Autodesk Inventor part; units mm, degrees
ref_plane "YZ Plane" through (0, 0, 0) normal (1, 0, 0) x (0, 1, 0)
ref_plane "XZ Plane" through (0, 0, 0) normal (0, 1, 0) x (-1, 0, 0)
ref_plane "XY Plane" through (0, 0, 0) normal (0, 0, 1) x (1, 0, 0)
sketch "Sketch1" plane through (0, 0, 0) normal (0, 1, 0) x (-1, 0, 0)
  line L0 (0, 0) -> (-2, 0)
  line L1 (-2, 0) -> (-2, 40)
  line L2 (-2, 40) -> (0, 40)
  line L3 (0, 40) -> (0, 0)
  line L4 (0, 0) -> (-42, 0)
  line L5 (-42, 0) -> (-42, -2)
  line L6 (-42, -2) -> (0, -2)
  line L7 (0, -2) -> (0, 0)
  dimension "d0" = 2
  dimension "d1" = 40
  dimension "d2" = 42
  dimension "d3" = 2
extrude "Extrusion1" add sketch "Sketch1" along normal blind 30
sketch "Sketch2" plane through (2, 0, 0) normal (0, 0, 1) x (1, 0, 0)
  line L0 (40.0406, 0) -> (40, 14.9999)
  line L1 (40, 0) -> (40, 30)
  line L2 (40, 14.9999) -> (29, 14.9702)
  line L3 (29, 14.9702) -> (12.0001, 14.9242)
  point P0 (-2, 0)
  dimension "d6" = 15
  dimension "d7" = 11
  dimension "d8" = 17
hole "Hole1" at (31, 14.9702, 0) at (14.0001, 14.9242, 0) direction (0, 0, -1) diameter 6 end through all
sketch "Sketch3" plane through (2, 0, 40) normal (1, 0, 0) x (0, 0, -1)
  line L0 (0, 0) -> (0, 30)
  line L1 (0, 0) -> (0, 15)
  line L2 (0, 15) -> (11, 15)
  line L3 (11, 15) -> (28, 15)
  point P0 (40, 0)
  dimension "d16" = 15
  dimension "d17" = 11
  dimension "d18" = 17
hole "Hole2" at (2, 15, 29) at (2, 15, 12) direction (-1, 0, 0) diameter 6 end through all
properties part number "3030_L-Bracket" material "Aluminum 6061"
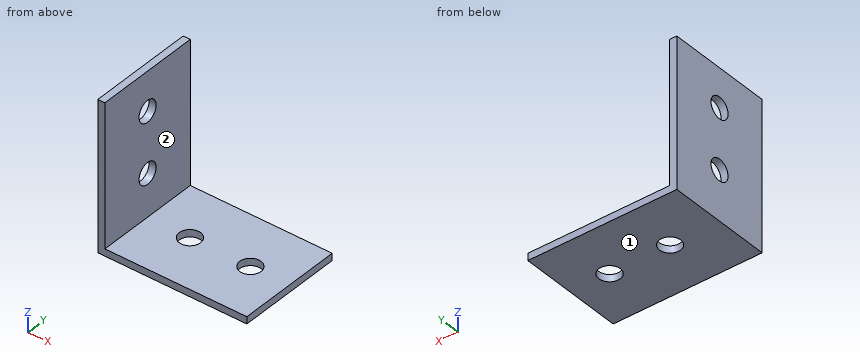
Here's how the part is built. I have some questions about the finished solid (model axes, mm). Face numbers are marked on the shaded views. A direction names the side the tool comes from. Give positions to 0.01 mm unless a question says otherwise; leave off trailing zeros. Loops run counter-clockwise (first coordinate to the right, second up) from the corner with the lowest first, then second, coordinate; pieces in that order, holes last. Notation, with made-up numbers: M 67,-38 L 113,-38 A27 ccw 113,-12 Z; hole C -28.75,-30.75 d11. An arc over 180 degrees is marked long. Use one line per item in the form item = value. Start each with the question number.
Q1. If we section it at A-A (z = 29): Write out the boundary of the cut face in (x, y).
Q2. If we section it at C-C (y = 2.75): Write out the boundary of the cut face in (x, z), then the cut area to 3 significant figures.
Q3. If we section it at B-B (x = 31): Write out the boundary of the cut face in (y, z), then the cut area to 3 significant figures.
Q4. Will these pins go through, and if not, where does the flat tip stop? pin 1 Ø12 at (x, y) = (14.5, 8.5) entering from +Z; pin 2 Ø2 at (y, z) = (11.5, 31.5) entering from -X; pin 3 Ø5 at (x, y) = (31, 14.97) entering from -Z; pin 4 Ø10 at (y, z) = (9.5, 15.5) entering from +X.
Q5. Which directions (+Z, -Z, +X, -X, +Y, -Y) give clear straight access to the entire face, cutting with the end or side of a thin tool? Please do the marked faces 1 and 2.
Q6. If we section it at D-D (y = 16.75): Write out the boundary of the cut face in (x, z).
Q7. I need wall thicknesses on line 1 along Z through (x, y) = (1.15, 15); line 2 along X through (y, z) = (16.5, 18.5); line 3 along Y through (x, z) = (31, -1). Which ranges of each line are inside material? Lowest first, please.
Taken from the geometry:
q1.outline = M 0,0 L 2,0 L 2,12 L 0,12 Z; M 0,18 L 2,18 L 2,30 L 0,30 Z
q2.outline = M 0,-2 L 42,-2 L 42,0 L 2,0 L 2,40 L 0,40 Z
q2.area = 164 mm^2
q3.outline = M 0,-2 L 11.97,-2 L 11.97,0 L 0,0 Z; M 17.97,-2 L 30,-2 L 30,0 L 17.97,0 Z
q3.area = 48.0 mm^2
q4.pin_1 = 0
q4.pin_2 = 0
q4.pin_3 = through
q4.pin_4 = 2
q5.face_1 = -Z, +X, -X, +Y, -Y
q5.face_2 = +Z, +X, +Y, -Y
q6.outline = M 0,-2 L 11.62,-2 L 11.62,0 L 2,0 L 2,9.56 L 0,9.56 Z; M 0,14.44 L 2,14.44 L 2,26.56 L 0,26.56 Z; M 0,31.44 L 2,31.44 L 2,40 L 0,40 Z; M 16.38,-2 L 28.58,-2 L 28.58,0 L 16.38,0 Z; M 33.42,-2 L 42,-2 L 42,0 L 33.42,0 Z
q7.line_1 = -2 to 9, 15 to 26, 32 to 40
q7.line_2 = 0 to 2
q7.line_3 = 0 to 11.97, 17.97 to 30
